Design review of the part built by this model. Coordinates are the model's own, in mm. A direction names the side the tool comes from. Round coordinates to 2 decimals unless told otherwise and drop trailing zeros. Loops run counter-clockwise (first coordinate to the right, second up) from the corner with the lowest first, then second, coordinate; pieces in that order, holes last. Notation, with made-up numbers: (47, 25.25) - (94, 25.25) arc R36 ccw to (94, 62.25) - close; hole circle Ø3 at (-7.5, 63.25). An arc over 180 degrees is marked (long way). Use one line per item in the form item = value. Start each with the question number.
(1) For pin 1 (6 mm diameter, centred on x = -2.31, z = 5.33, fed in from -Y); pin 2 (2 mm diameter, centred on x = -53, y = -8.5, fed in from -Z); pin 3 (8.5 mm diameter, centred on x = -51, z = 6, fed in from +Y), all flat-tipped, find the tip position at first contact; note any pin that passes through.
(2) Wall thickness on probe 1 along X at (y, z) = (-7.5, 16.25); probe 2 along X at (y, z) = (-0.5, 13.5); probe 3 along Y at (x, z) = (-31, 13.5): over which ranges is each line inside the solid? List them lowest first. Write a range as [from, to].
(3) We need section A-A, the plane z = 6. Write out the cut boundary in (x, y), then the cut area to 3 significant figures.
(4) We need section B-B, the plane z = 2. Write out the cut boundary in (x, y), then the cut area to 3 significant figures.
(5) We need section C-C, the plane x = -31. Write out the cut boundary in (y, z).
(6) The part is to be moulded in two halves that separate along Z. For faces 1 (the flat face through (-4, -8, 18.961)), 2 (the cylindrical face through (-1.29, -8.38, 7.3)), 3 (the cylindrical face through (-34.516, 2.824, 9.009)), 4 (the flat face through (-28, -35.966, 10)), say which applies: released by +Z, released by -Z, zero draft, split by the parting line, or undercut.
(7) We need section D-D, the plane y = -12.5. Write out the cut boundary in (x, z), then the cut area to 3 significant figures.
(8) Machinability: for faces 5 (the flat face through (-5, -7.163, 10)), 6 (the flat face through (-51, -9.627, 10)), 7 (the flat face through (-51, -7.163, 10)), 8 (the flat face through (-52, -8, 0.902)), which of the approach directions +Z, -Z, +X, -X, +Y, -Y give a long, thin tool a straight path to every point of the face, cutting with its end or side? Answer none if there is none.
from build123d import *

# Parameters (mm, degrees)
SKETCH1_W           = 55.499
SKETCH1_H           = 35.9664
BOSS_EXTRUDE1_DEPTH = 19.8628
SKETCH2_W           = 7.7216
SKETCH2_H           = 7.1628
SKETCH2_H_2         = 26.3398
CUT_EXTRUDE1_DEPTH  = 19.8628
SKETCH3_W           = 7.7216
SKETCH3_H           = 7.1628
SKETCH3_H_2         = 26.3398
CUT_EXTRUDE2_DEPTH  = 19.8628
SKETCH4_R           = 2.21615
CUT_EXTRUDE3_DEPTH  = 2.4638
SKETCH5_W           = 7.7216
SKETCH5_H           = 2.4638
CUT_EXTRUDE4_DEPTH  = 0.9017
SKETCH6_W           = 7.7216
SKETCH6_H           = 2.4638
CUT_EXTRUDE5_DEPTH  = 0.9017
SKETCH7_W           = 7.7216
SKETCH7_H           = 2.4638
CUT_EXTRUDE6_DEPTH  = 0.9017
SKETCH8_W           = 7.7216
SKETCH8_H           = 2.4638
CUT_EXTRUDE7_DEPTH  = 0.9017
SKETCH9_R           = 2.96545
BOSS_EXTRUDE2_DEPTH = 5.7277


with BuildPart() as part:
    # Sketch1 → Boss-Extrude1 (new body)
    with BuildSketch(Plane.XY):
        with Locations((-27.7495, -17.9832)):
            Rectangle(SKETCH1_W, SKETCH1_H)
    extrude(amount=BOSS_EXTRUDE1_DEPTH)

    # Sketch2 → Cut-Extrude1 (cut)
    with BuildSketch(Plane.XY.offset(19.8628)):
        with Locations((-51.6382, -3.5814)):
            Rectangle(SKETCH2_W, SKETCH2_H)
        with Locations((-51.6382, -22.7965)):
            Rectangle(SKETCH2_W, SKETCH2_H_2)
    extrude(amount=-CUT_EXTRUDE1_DEPTH, mode=Mode.SUBTRACT)

    # Sketch3 → Cut-Extrude2 (cut)
    with BuildSketch(Plane.XY.offset(19.8628)):
        with Locations((-3.8608, -3.5814)):
            Rectangle(SKETCH3_W, SKETCH3_H)
        with Locations((-3.8608, -22.7965)):
            Rectangle(SKETCH3_W, SKETCH3_H_2)
    extrude(amount=-CUT_EXTRUDE2_DEPTH, mode=Mode.SUBTRACT)

    # Sketch4 → Cut-Extrude3 (cut)
    with BuildSketch(Plane(origin=(0, -7.1628, 0), x_dir=(1, 0, 0), z_dir=(0, 1, 0))):
        with Locations((-53.14315, -5.26415)):
            Circle(SKETCH4_R)
        with Locations((-53.14315, -15.15745)):
            Circle(SKETCH4_R)
        with Locations((-2.314703143, -5.334451514)):
            Circle(SKETCH4_R)
        with Locations((-2.314703143, -15.227751514)):
            Circle(SKETCH4_R)
    extrude(amount=-CUT_EXTRUDE3_DEPTH, mode=Mode.SUBTRACT)

    # Sketch5 → Cut-Extrude4 (cut)
    with BuildSketch(Plane.XY.offset(19.8628)):
        with Locations((-51.6382, -8.3947)):
            Rectangle(SKETCH5_W, SKETCH5_H)
    extrude(amount=-CUT_EXTRUDE4_DEPTH, mode=Mode.SUBTRACT)

    # Sketch6 → Cut-Extrude5 (cut)
    with BuildSketch(Plane(origin=(0, 0, 0), x_dir=(-1, 0, 0), z_dir=(0, 0, -1))):
        with Locations((51.6382, -8.3947)):
            Rectangle(SKETCH6_W, SKETCH6_H)
    extrude(amount=-CUT_EXTRUDE5_DEPTH, mode=Mode.SUBTRACT)

    # Sketch7 → Cut-Extrude6 (cut)
    with BuildSketch(Plane(origin=(0, 0, 0), x_dir=(-1, 0, 0), z_dir=(0, 0, -1))):
        with Locations((3.8608, -8.3947)):
            Rectangle(SKETCH7_W, SKETCH7_H)
    extrude(amount=-CUT_EXTRUDE6_DEPTH, mode=Mode.SUBTRACT)

    # Sketch8 → Cut-Extrude7 (cut)
    with BuildSketch(Plane.XY.offset(19.8628)):
        with Locations((-3.8608, -8.3947)):
            Rectangle(SKETCH8_W, SKETCH8_H)
    extrude(amount=-CUT_EXTRUDE7_DEPTH, mode=Mode.SUBTRACT)

    # Sketch9 → Boss-Extrude2 (add)
    with BuildSketch(Plane(origin=(0, 0, 0), x_dir=(1, 0, 0), z_dir=(0, 1, 0))):
        with Locations((-37.34435, -9.89965)):
            Circle(SKETCH9_R)
    extrude(amount=BOSS_EXTRUDE2_DEPTH)


solid = part.part
Data:
q1.pin_1 = -9.63
q1.pin_2 = 0.9
q1.pin_3 = 0
q2.probe_1 = [-55.5, -55.07], [-51.22, -4.28], [-0.35, 0]
q2.probe_2 = [-47.78, -7.72]
q2.probe_3 = [-35.97, 0]
q3.outline = (-55.5, -9.63) - (-55.23, -9.63) - (-55.23, -7.16) - (-55.5, -7.16) - close; (-51.05, -9.63) - (-47.78, -9.63) - (-47.78, -35.97) - (-7.72, -35.97) - (-7.72, -9.63) - (-4.43, -9.63) - (-4.43, -7.16) - (-7.72, -7.16) - (-7.72, 0) - (-47.78, 0) - (-47.78, -7.16) - (-51.05, -7.16) - close; (-0.2, -9.63) - (0, -9.63) - (0, -7.16) - (-0.2, -7.16) - close
q3.area = 1,460 mm^2
q4.outline = (-55.5, -9.63) - (-47.78, -9.63) - (-47.78, -35.97) - (-7.72, -35.97) - (-7.72, -9.63) - (0, -9.63) - (0, -7.16) - (-7.72, -7.16) - (-7.72, 0) - (-47.78, 0) - (-47.78, -7.16) - (-55.5, -7.16) - close
q4.area = 1,480 mm^2
q5.outline = (-35.97, 0) - (0, 0) - (0, 19.86) - (-35.97, 19.86) - close
q6.face_1 = released by +Z
q6.face_2 = undercut
q6.face_3 = split by the parting line
q6.face_4 = zero draft
q7.outline = (-47.78, 0) - (-7.72, 0) - (-7.72, 19.86) - (-47.78, 19.86) - close
q7.area = 796 mm^2
q8.face_5 = +Z, -Z, +X, +Y
q8.face_6 = +Z, -Z, -X, -Y
q8.face_7 = +Z, -Z, -X, +Y
q8.face_8 = -Z, -X, +Y, -Y
